Input: dimensioned drawing with shaded views. Units: mm. Origin: part minimum x, y, z. A direction names the side the tool comes from. Coordinates: 2 decimals unless noted, no trailing zeros. Loops run counter-clockwise (first coordinate to the right, second up) from the corner with the lowest first, then second, coordinate; pieces in that order, holes last. Notation, with made-up numbers: (72, 49) - (93, 49) arc R26 cw to (93, 65) - close; hole circle Ø3 at (52.5, 25). An arc over 180 degrees is marked (long way). Put each result on its own line as item: value. Start each with the question number.
1) Section B-B on x = 64. Output: boundary loops of the cut face in (y, z), and give its area (3 significant figures).
2) Reachability of the marked faces 5, 6 and 7 from +Z, -Z, +X, -X, +Y, -Y: full face, straight path, thin tool, end or side. Return the list, or none.
3) Section C-C on z = 1.75. Output: boundary loops of the cut face in (x, y), and give its area (3 significant figures).
4) Section A-A on y = 17.5. Output: boundary loops of the cut face in (x, z), and give its area (3 significant figures).
5) Draft query along X for the marked faces 1, 2, 3 and 4. Return one class per face: +X half, -X half, draft (parallel to the pull), parting line (faces both ways), or undercut.
6) Section D-D on y = 4. Output: boundary loops of the cut face in (x, z), and give its area (4 significant figures).
7) Material intervals for line 1 along Y through (x, z) = (40, 7.5); line 2 along Y through (x, z) = (69.5, 5); line 3 along X through (y, z) = (20, 10.5), sorted ascending. Write a range as from..to.
8) Contact query for flat-ended pins moving along their axis: pin 1 Ø6 at (y, z) = (13, 13) entering from +X; pin 2 Ø3.5 at (y, z) = (19.5, 9) entering from -X; pin 3 Ø6 at (y, z) = (18, 8.5) entering from +X. Output: stop coordinate, or through.
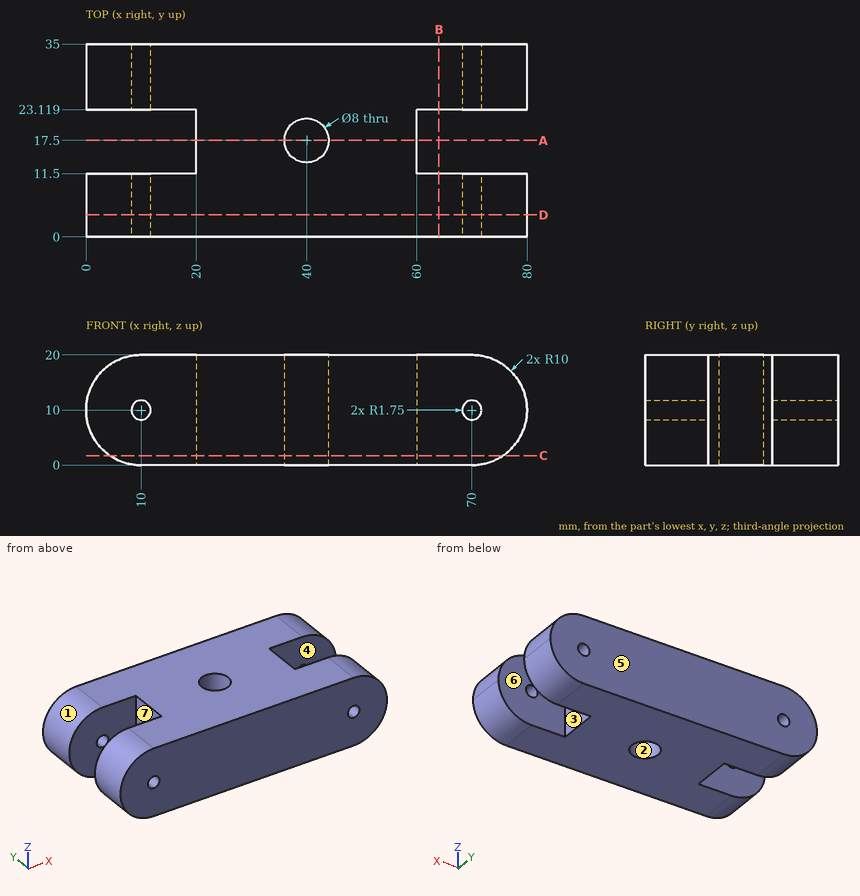
Answer block:
1. outline: (0, 0) - (11.5, 0) - (11.5, 20) - (0, 20) - close; (23.12, 0) - (35, 0) - (35, 20) - (23.12, 20) - close
1. area: 468 mm²
2. face 5: +Z, -Z, +X, -X, +Y
2. face 6: +Z, -Z, +X
2. face 7: +Z, -Z, -X
3. outline: (4.35, 0) - (75.65, 0) - (75.65, 11.5) - (60, 11.5) - (60, 23.12) - (75.65, 23.12) - (75.65, 35) - (4.35, 35) - (4.35, 23.12) - (20, 23.12) - (20, 11.5) - (4.35, 11.5) - close; hole circle Ø8 at (40, 17.5)
3. area: 2,080 mm²
4. outline: (20, 0) - (36, 0) - (36, 20) - (20, 20) - close; (44, 0) - (60, 0) - (60, 20) - (44, 20) - close
4. area: 640 mm²
5. face 1: -X half
5. face 2: undercut
5. face 3: +X half
5. face 4: draft
6. outline: (10, 0) - (70, 0) arc R10 ccw to (70, 20) - (10, 20) arc R10 ccw to start; hole circle Ø3.5 at (10, 10); hole circle Ø3.5 at (70, 10)
6. area: 1,495 mm²
7. line 1: y = 0..13.5, 21.5..35
7. line 2: y = 0..11.5, 23.12..35
7. line 3: x = 20..36.88, 43.12..60
8. pin 1: stops at x = 79.99
8. pin 2: stops at x = 20
8. pin 3: stops at x = 60
